from build123d import *

# Parameters (mm, degrees)
SKETCH_1_R          = 2.5
EXTRUDE_1_DEPTH     = 2
SKETCH_2_R          = 2.000656811
SKETCH_2_R_2        = 2.054404912
SKETCH_2_R_3        = 2
SKETCH_2_R_4        = 1.847510468
CUT_EXTRUDE_1_DEPTH = 3


with BuildPart() as part:
    # 草图1 → 凸台-拉伸1 (new body)
    with BuildSketch(Plane(origin=(0, 0, 0), x_dir=(0, 0, -1), z_dir=(1, 0, 0))):
        with BuildLine():
            Line((80, -100), (-80, -100))
            Line((-80, -100), (-80, 100))
            Line((-80, 100), (-80, 117.438447187))
            Line((-80, 117.438447187), (-80, 120))
            Line((-80, 120), (-77.51492875, 119.378732187))
            Line((-77.51492875, 119.378732187), (-5.971499971, 101.492874993))
            ThreePointArc((-5.971499971, 101.492874993), (0.046118096, 100.374622166), (6.155281281, 100))
            Line((6.155281281, 100), (80, 100))
            Line((80, 100), (80, -100))
        make_face()
        with Locations((-65.5, -10)):
            Circle(SKETCH_1_R, mode=Mode.SUBTRACT)
        with Locations((-33.5, -10)):
            Circle(SKETCH_1_R, mode=Mode.SUBTRACT)
        with Locations((-65.5, 85)):
            Circle(SKETCH_1_R, mode=Mode.SUBTRACT)
        with Locations((-33.5, 85)):
            Circle(SKETCH_1_R, mode=Mode.SUBTRACT)
        with Locations((33.5, 85)):
            Circle(SKETCH_1_R, mode=Mode.SUBTRACT)
        with Locations((65.5, 85)):
            Circle(SKETCH_1_R, mode=Mode.SUBTRACT)
        with Locations((33.5, -10)):
            Circle(SKETCH_1_R, mode=Mode.SUBTRACT)
        with Locations((65.5, -10)):
            Circle(SKETCH_1_R, mode=Mode.SUBTRACT)
        with Locations((0, -91)):
            Circle(SKETCH_1_R, mode=Mode.SUBTRACT)
        with Locations((-15.25, -71.5)):
            Circle(SKETCH_1_R, mode=Mode.SUBTRACT)
        with Locations((15.25, -71.5)):
            Circle(SKETCH_1_R, mode=Mode.SUBTRACT)
    extrude(amount=EXTRUDE_1_DEPTH)

    # 草图2 → 切除-拉伸1 (cut, through all)
    with BuildSketch(Plane(origin=(2, 0, 0), x_dir=(0, 0, -1), z_dir=(1, 0, 0))):
        with Locations((68.472742663, 37.640760233)):
            Circle(SKETCH_2_R)
        with Locations((39.073599545, 35.20346994)):
            Circle(SKETCH_2_R_2)
        with Locations((-21.219558373, 30.20495934)):
            Circle(SKETCH_2_R_3)
        with Locations((4.495464774, -37.903319045)):
            Circle(SKETCH_2_R_4)
    extrude(amount=-CUT_EXTRUDE_1_DEPTH, mode=Mode.SUBTRACT)


solid = part.part
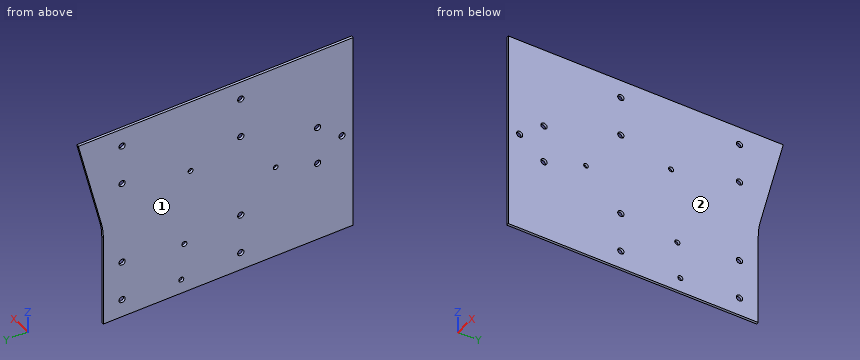
Could you check a few things on this model? Use its own coordinates, in mm. Face numbers are marked on the shaded views. Give positions to 0.01 mm unless a question says otherwise; leave off trailing zeros. Order: outer loops, then holes, each group sorted by start corner. A loop starts at its lowest first (then second) coordinate and runs counter-clockwise, first axis right, second up. Notation, with made-up numbers: (40, -16) - (77, -16) arc R16 ccw to (77, 8) - close; hole circle Ø8 at (76, 56). An arc over 180 degrees is marked (long way). One line per question, with ' | ' between items. Start each with the question number.
Item 1: I want a section at D-D on z = 65.5. Write out the boundary of the cut face in (x, y) (3 decimals).
Item 2: I need wall thicknesses on probe 1 along Y at (x, z) = (0.75, -65.5); probe 2 along Y at (x, z) = (1.95, -4.5); probe 3 along Y at (x, z) = (1.7, 34.5) (3 decimals). Which ranges of each line are inside material? Lowest first, please. Write a range as [from, to].
Item 3: I want a section at C-C on y = -91. Write out the boundary of the cut face in (x, z).
Item 4: I want a section at B-B on z = -15.25. Write out the boundary of the cut face in (x, y).
Item 5: Thinking about a two-plate mould opening in X: for the marked faces 1 and 2, which applies, pulls with the +X half, pulls with the -X half, needs draft (parallel to the pull), parting line crosses it, or undercut?
Item 6: I want a section at A-A on y = -10. Write out the boundary of the cut face in (x, z), then the cut area to 3 significant figures.
Item 7: I'm going to push a flat-ended pin straight in: pin 1 Ø3 at (y, z) = (-71.5, -15.25) entering from -X. Where does the tip first touch, or does it pass through?
Verdict:
1) outline: (0, -100) - (2, -100) - (2, -12.5) - (0, -12.5) - close; (0, -7.5) - (2, -7.5) - (2, 82.5) - (0, 82.5) - close; (0, 87.5) - (2, 87.5) - (2, 116.375) - (0, 116.375) - close
2) probe 1: [-100, -12.5], [-7.5, 82.5], [87.5, 100] | probe 2: [-100, -39.75], [-36.06, 100.03] | probe 3: [-100, -12.291], [-7.709, 82.709], [87.291, 108.625]
3) outline: (0, -80) - (2, -80) - (2, -2.5) - (0, -2.5) - close; (0, 2.5) - (2, 2.5) - (2, 80) - (0, 80) - close
4) outline: (0, -100) - (2, -100) - (2, -74) - (0, -74) - close; (0, -69) - (2, -69) - (2, 100) - (0, 100) - close
5) face 1: pulls with the -X half | face 2: pulls with the +X half
6) outline: (0, -80) - (2, -80) - (2, -68) - (0, -68) - close; (0, -63) - (2, -63) - (2, -36) - (0, -36) - close; (0, -31) - (2, -31) - (2, 31) - (0, 31) - close; (0, 36) - (2, 36) - (2, 63) - (0, 63) - close; (0, 68) - (2, 68) - (2, 80) - (0, 80) - close | area: 280 mm^2
7) pin 1: through
